Verification items for the finished model (mm, model axes). A direction names the side the tool comes from. Round coordinates to 2 decimals unless told otherwise and drop trailing zeros. Loops run counter-clockwise (first coordinate to the right, second up) from the corner with the lowest first, then second, coordinate; pieces in that order, holes last. Notation, with made-up numbers: (-5, 21) -> (49, 21) arc R26 cw to (49, 42) -> close; hole circle Ø9 at (-34.75, 23.5). An arc over 180 degrees is marked (long way). Write item = value, one per line.
```python
from build123d import *

# Parameters (mm, degrees)
SKETCH1_W                                         = 304.8
SKETCH1_H                                         = 254
BOSS_EXTRUDE1_DEPTH                               = 6.35
SKETCH2_W                                         = 228.6
SKETCH2_H                                         = 177.8
CUT_EXTRUDE1_DEPTH                                = 6.35
FILLET1_R                                         = 2.54
FILLET5_R                                         = 12.7
SKETCH6_W                                         = 12.7
SKETCH6_H                                         = 3.81
BOSS_EXTRUDE3_DEPTH                               = 21.59
SKETCH8_R                                         = 1.905
CUT_EXTRUDE5_DEPTH                                = 12.7
CSK_FOR_8_FLAT_HEAD_MACHINE_SCREW_100_D           = 4.9149
CSK_FOR_8_FLAT_HEAD_MACHINE_SCREW_100_DEPTH       = 10.668
CSK_FOR_8_FLAT_HEAD_MACHINE_SCREW_100_CSINK_D     = 8.4328
CSK_FOR_8_FLAT_HEAD_MACHINE_SCREW_100_CSINK_ANGLE = 100
CSK_FOR_8_FLAT_HEAD_MACHINE_SCREW_100_TIP         = 1.476584928


with BuildPart() as part:
    # Sketch1 → Boss-Extrude1 (new body)
    with BuildSketch(Plane(origin=(0, 0, 0), x_dir=(1, 0, 0), z_dir=(0, 1, 0))):
        Rectangle(SKETCH1_W, SKETCH1_H)
    extrude(amount=BOSS_EXTRUDE1_DEPTH)

    # Sketch2 → Cut-Extrude1 (cut)
    with BuildSketch(Plane(origin=(0, 6.35, 0), x_dir=(1, 0, 0), z_dir=(0, 1, 0))):
        Rectangle(SKETCH2_W, SKETCH2_H)
    extrude(amount=-CUT_EXTRUDE1_DEPTH, mode=Mode.SUBTRACT)

    # Fillet1
    fillet1_edges = [part.edges().sort_by_distance(p)[0] for p in [
        (114.3, 6.35, 0),
        (0, 6.35, -88.9),
        (-114.3, 6.35, 0),
        (0, 6.35, 88.9),
    ]]
    fillet(fillet1_edges, radius=FILLET1_R)

    # Fillet5
    fillet5_edges = [part.edges().sort_by_distance(p)[0] for p in [
        (152.4, 3.175, 127),
        (-152.4, 3.175, 127),
        (-152.4, 3.175, -127),
        (152.4, 3.175, -127),
    ]]
    fillet(fillet5_edges, radius=FILLET5_R)

    # Sketch6 → Boss-Extrude3 (add)
    with BuildSketch(Plane.XZ):
        with Locations((-120.65, 0)):
            Rectangle(SKETCH6_W, SKETCH6_H)
    boss_extrude3 = extrude(amount=BOSS_EXTRUDE3_DEPTH)

    # Sketch8 → Cut-Extrude5 (cut)
    with BuildSketch(Plane.ZY.offset(127)):
        with Locations((0, -21.59)):
            Circle(SKETCH8_R)
    cut_extrude5 = extrude(amount=-CUT_EXTRUDE5_DEPTH, mode=Mode.SUBTRACT)

    # Mirror1: Boss-Extrude3, Cut-Extrude5 across plane
    add(boss_extrude3.mirror(Plane(origin=(0, 0, 0), x_dir=(0, 0, 1), z_dir=(1, 0, 0))))
    add(cut_extrude5.mirror(Plane(origin=(0, 0, 0), x_dir=(0, 0, 1), z_dir=(1, 0, 0))), mode=Mode.SUBTRACT)

    # CSK for #8 Flat Head Machine Screw (100)1
    with Locations(Plane(origin=(0, 6.35, 0), x_dir=(1, 0, 0), z_dir=(0, 1, 0))):
        with Locations((-139.7, -114.3), (139.7, -114.3), (139.7, 114.3), (-139.7, 114.3)):
            CounterSinkHole(CSK_FOR_8_FLAT_HEAD_MACHINE_SCREW_100_D / 2, CSK_FOR_8_FLAT_HEAD_MACHINE_SCREW_100_CSINK_D / 2, depth=CSK_FOR_8_FLAT_HEAD_MACHINE_SCREW_100_DEPTH, counter_sink_angle=CSK_FOR_8_FLAT_HEAD_MACHINE_SCREW_100_CSINK_ANGLE)
            with Locations((0, 0, -(CSK_FOR_8_FLAT_HEAD_MACHINE_SCREW_100_DEPTH + CSK_FOR_8_FLAT_HEAD_MACHINE_SCREW_100_TIP / 2))):  # 118° drill point
                Cone(0, CSK_FOR_8_FLAT_HEAD_MACHINE_SCREW_100_D / 2, CSK_FOR_8_FLAT_HEAD_MACHINE_SCREW_100_TIP, mode=Mode.SUBTRACT)


solid = part.part
```
(1) Sectioned sample at A-A, the plane x = 80. Record the cut outline in (y, z), and give its area (3 significant figures).
Filled sheet:
outline = (0, -127) -> (6.35, -127) -> (6.35, -91.44) arc R2.54 ccw to (3.81, -88.9) -> (0, -88.9) -> close; (0, 88.9) -> (3.81, 88.9) arc R2.54 ccw to (6.35, 91.44) -> (6.35, 127) -> (0, 127) -> close
area = 481 mm2
(2) Material ranges on probe 1 along Z at (x, y) = (-139.7, 1.6); probe 2 along X at (y, z) = (1.7, -114.3); probe 3 along Z at (x, y) = (105, 1), recorded low to high. Write a range as from..to.
Filled sheet:
probe_1 = -127..-116.76, -111.84..111.84, 116.76..127
probe_2 = -152.4..-142.16, -137.24..137.24, 142.16..152.4
probe_3 = -127..-88.9, 88.9..127
(3) Sectioned sample at B-B, the plane y = -14. Record the cut outline in (x, z) (3 decimals), and give its area (3 significant figures).
Filled sheet:
outline = (-127, -1.905) -> (-114.3, -1.905) -> (-114.3, 1.905) -> (-127, 1.905) -> close; (114.3, -1.905) -> (127, -1.905) -> (127, 1.905) -> (114.3, 1.905) -> close
area = 96.8 mm2
(4) Draft check along Z on faces 1 (the face through (-148.78, 3.22, 123.18)), 2 (the face through (152.4, 3, 2)), 3 (the face through (-114.3, 1, 0)). Enter one of: released by +Z, released by -Z, zero draft, split by the parting line, or undercut.
Filled sheet:
face_1 = released by +Z
face_2 = zero draft
face_3 = undercut
(5) Sectioned sample at C-C, the plane z = 13. Record the cut outline in (x, y).
Filled sheet:
outline = (-152.4, 0) -> (-114.3, 0) -> (-114.3, 3.81) arc R2.54 ccw to (-116.84, 6.35) -> (-152.4, 6.35) -> close; (114.3, 0) -> (152.4, 0) -> (152.4, 6.35) -> (116.84, 6.35) arc R2.54 ccw to (114.3, 3.81) -> close
(6) Set-up check for faces 4 (the face through (121, -11, 1.905)), 5 (the face through (-121, -11, -1.905)), 6 (the face through (114.3, 1, 0)): record each of +Z, -Z, +X, -X, +Y, -Y from which the full face is reachable in a straight line by a thin tool's end or side.
Filled sheet:
face_4 = +Z, +X, -X, -Y
face_5 = -Z, +X, -X, -Y
face_6 = +Y, -Y
(7) Go/stop test with flat-tipped pins: pin 1 Ø1.9 at (y, z) = (-10.5, -0.5) entering from -X; pin 2 Ø14 at (x, y) = (-120, -13) entering from -Z (3 decimals); pin 3 Ø1.1 at (y, z) = (-6.5, 0.5) entering from +X. Record where each tip stops, or that it passes through.
Filled sheet:
pin_1 = -127
pin_2 = -1.905
pin_3 = 127
(8) Sectioned sample at D-D, the plane x = -122. Record the cut outline in (y, z) (3 decimals), and give its area (3 significant figures).
Filled sheet:
outline = (-21.59, -1.905) -> (0, -1.905) -> (0, -127) -> (6.35, -127) -> (6.35, 127) -> (0, 127) -> (0, 1.905) -> (-21.59, 1.905) arc R1.905 cw to start
area = 1,690 mm2
